from build123d import *

# Parameters (mm, degrees)
SKETCH_R      = 9.125
PAD_DEPTH     = 2
SKETCH001_R   = 9.125
SKETCH001_R_2 = 7.125
PAD001_DEPTH  = 7
CHAMFER_SIZE  = 1.5
FILLET_R      = 1


with BuildPart() as part:
    # Sketch → Pad (new body)
    with BuildSketch(Plane.XY):
        Circle(SKETCH_R)
    extrude(amount=PAD_DEPTH)

    # Sketch001 (on Face3 of Pad) → Pad001 (join)
    with BuildSketch(Plane.XY.offset(2)):
        Circle(SKETCH001_R)
        Circle(SKETCH001_R_2, mode=Mode.SUBTRACT)
    extrude(amount=PAD001_DEPTH)

    # Chamfer
    chamfer_edges = [part.edges().sort_by_distance(p)[0] for p in [
        (-7.125, 0, 9),
    ]]
    chamfer(chamfer_edges, length=CHAMFER_SIZE)

    # Fillet
    fillet_edges = [part.edges().sort_by_distance(p)[0] for p in [
        (-7.125, 0, 7.5),
    ]]
    fillet(fillet_edges, radius=FILLET_R)


solid = part.part
Work out the finished part from the listing and answer in its coordinate system (mm). Coordinates: 2 decimals unless noted, no trailing zeros. Write each loop counter-clockwise with the first axis right and the second up, starting at its lowest first coordinate (ties: lowest second). Pieces come first, ordered by that corner, then holes. Notation, with made-up numbers: M -37,61 L -31,61 A28 cw -31,99 Z; hole C 25,19 d6. An arc over 180 degrees is marked long. Answer as CSV lines item,"result". Start each with the question number.
Item 1: Determine the mould class of faces 1 (the face through (-1.978, -8.908, 4.437)), 2 (the face through (0, 0, 2)), 3 (the face through (0, 0, 0)) for opening direction X: released by +X, released by -X, zero draft, split by the parting line, or undercut.
Item 2: Section B-B on z = 0.75 is taken. Write down the section's boundary in (x, y) (3 decimals), and give its area (3 significant figures).
Item 3: Consider L1, parallel to Y at x = 0, z = 5.2 (3 decimals); L2, parallel to Z at x = 4.25, y = -2; L3, parallel to Y at x = 3.5, z = 4.75. Determine where each line is inside the solid, lowest interval first.
Item 4: Section A-A on z = 6.5 is taken. Write down the section's boundary in (x, y) (3 decimals), and give its area (3 significant figures).
Item 5: Flat-ended cylindrical pins translate along their axes: P1, Ø1.5, axis at x = 2, y = -5, coming from the +Z side; P2, Ø2, axis at x = -2.5, z = 3, coming from the -Y side; P3, Ø1, axis at x = -1, z = 3, coming from the +Y side. Find the tip coordinate at first contact, or state that the pin passes through.
Checks:
1,face 1,"split by the parting line"
1,face 2,"undercut"
1,face 3,"zero draft"
2,outline,"C 0,0 d18.25"
2,area,"262 mm²"
3,L1,"y = -9.125 to -7.125, 7.125 to 9.125"
3,L2,"z = 0 to 2"
3,L3,"y = -8.43 to -6.21, 6.21 to 8.43"
4,outline,"C 0,0 d18.25; hole C 0,0 d14.25"
4,area,"102 mm²"
5,P1,"stops at z = 2"
5,P2,"stops at y = -9"
5,P3,"stops at y = 9.11"
